```python
from build123d import *

# Parameters (mm, degrees)
F0_R     = 30
F0_R_2   = 4
F1_DEPTH = 12
F2_R     = 2.25
F3_DEPTH = 2
F4_R     = 1.55
F5_DEPTH = 25
F6_R     = 3
F7_DEPTH = 6
F9_DEPTH = 2
F10_SIZE = 0.5


with BuildPart() as f1:
    # F0 (on Top) → F1 (new body)
    with BuildSketch(Plane.XY):
        Circle(F0_R)
        Circle(F0_R_2, mode=Mode.SUBTRACT)
    extrude(amount=F1_DEPTH)

    # F2 (on face) → F3 (cut)
    with BuildSketch(Plane.XY.offset(12)):
        with Locations((0, 11.425)):
            Circle(F2_R)
    extrude(amount=-F3_DEPTH, mode=Mode.SUBTRACT)

    # F4 (on face) → F5 (cut)
    with BuildSketch(Plane.XY.offset(12)):
        with Locations((8.7, 20.925)):
            Circle(F4_R)
        with Locations((-8.7, 20.925)):
            Circle(F4_R)
        with Locations((0, -13.7)):
            Circle(F4_R)
    extrude(amount=-F5_DEPTH, mode=Mode.SUBTRACT)

    # F6 (on face) → F7 (cut)
    with BuildSketch(Plane(origin=(0, 0, 0), x_dir=(1, 0, 0), z_dir=(0, 0, -1))):
        with Locations((0, 13.7)):
            Circle(F6_R)
        with Locations((-8.7, -20.925)):
            Circle(F6_R)
        with Locations((8.7, -20.925)):
            Circle(F6_R)
    extrude(amount=-F7_DEPTH, mode=Mode.SUBTRACT)

    # F8 (on face) → F9 (cut)
    with BuildSketch(Plane.XY.offset(12)):
        with BuildLine():
            Line((21.28461, 11.133975), (26.466324, 14.125639))
            ThreePointArc((26.466324, 14.125639), (25.980762, 15), (25.466324, 15.85769))
            Line((25.466324, 15.85769), (20.28461, 12.866025))
            Line((20.28461, 12.866025), (21.28461, 11.133975))
        make_face()
        with BuildLine():
            Line((1, -29.983329), (1, -24))
            Line((1, -24), (-1, -24))
            Line((-1, -24), (-1, -29.983329))
            ThreePointArc((-1, -29.983329), (0, -30), (1, -29.983329))
        make_face()
        with BuildLine():
            Line((-20.28461, 12.866025), (-25.466324, 15.85769))
            ThreePointArc((-25.466324, 15.85769), (-25.980762, 15), (-26.466324, 14.125639))
            Line((-26.466324, 14.125639), (-21.28461, 11.133975))
            Line((-21.28461, 11.133975), (-20.28461, 12.866025))
        make_face()
    extrude(amount=-F9_DEPTH, mode=Mode.SUBTRACT)

    # F10
    f10_edges = [f1.edges().sort_by_distance(p)[0] for p in [
        (-30, 0, 0),
        (-3, -13.7, 0),
        (-4, 0, 0),
        (-11.7, 20.925, 0),
        (5.7, 20.925, 0),
    ]]
    chamfer(f10_edges, length=F10_SIZE)


solid = f1.part
```
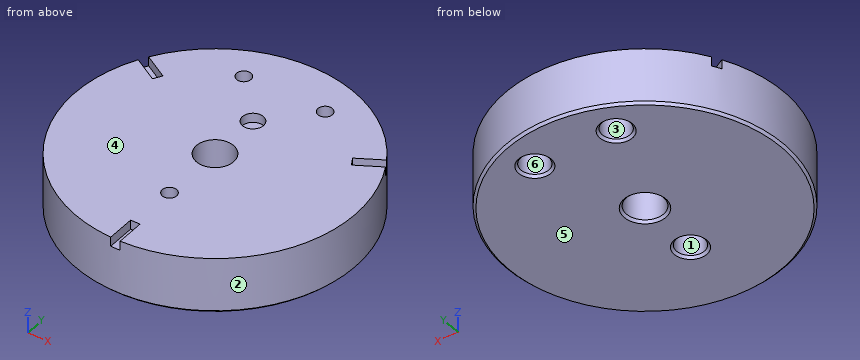
The listing builds one solid part. Answer for the finished solid, in the listing's coordinates (mm). Face numbers are marked on the shaded views. A direction names the side the tool comes from. Give positions to 0.01 mm unless a question says otherwise; leave off trailing zeros. Loops run counter-clockwise (first coordinate to the right, second up) from the corner with the lowest first, then second, coordinate; pieces in that order, holes last. Notation, with made-up numbers: (-16.75, -34) - (40.25, -34) arc R7 ccw to (40.25, -22) - close; hole circle Ø4 at (83.5, -35). An arc over 180 degrees is marked (long way). Return JSON: item names as keys, results as strings. Group by question number.
1. Find section C-C (z = 3.5). Write down the section's boundary in (x, y) (3 decimals), then the cut area to 3 significant figures.
2. Determine the mould class of the marked faces 1, 2, 3 and 4 for opening direction Y: pulls with the +Y half, pulls with the -Y half, needs draft (parallel to the pull), parting line crosses it, or undercut.
3. Given pin 1 Ø3 at (x, y) = (-10, 22) entering from -Z; pin 2 Ø0.6 at (x, y) = (0, -27.5) entering from +Z; pin 3 Ø4 at (x, y) = (23.5, 13.5) entering from +Z; pin 4 Ø1.5 at (x, z) = (-3.5, 2.5) entering from -Y, each flat-ended and moving along its own axis, determine where each tip first touches the part or whether it passes through.
4. Find section B-B (y = 0). Write down the section's boundary in (x, z).
5. Find section A-A (x = 0). Write down the section's boundary in (y, z) (3 decimals), then the cut area to 3 significant figures.
6. Which of the six approach directions +Z, -Z, +X, -X, +Y, -Y give full straight-line access (tool end or side, diameter ignored) to the marked faces 5 and 6?
7. Find section D-D (z = 8.75). Write down the section's boundary in (x, y) (3 decimals), then the cut area to 3 significant figures.
8. Straight lines are drawn through the part: line 1 (Y direction, x = 0, z = 5); line 2 (X direction, y = 20.5, z = 3.75); line 3 (X direction, y = -3.5, z = 1.25). For each, find the intervals that lie inside material, in ascending order. Write a range as [from, to].
Verdict:
{
 "1": {"outline": "circle Ø60 at (0, 0); hole circle Ø6 at (-8.7, 20.925); hole circle Ø8 at (0, 0); hole circle Ø6 at (0, -13.7); hole circle Ø6 at (8.7, 20.925)", "area": "2,690 mm^2"},
 "2": {"face 1": "undercut", "face 2": "parting line crosses it", "face 3": "undercut", "face 4": "needs draft"},
 "3": {"pin 1": "stops at z = 0.31", "pin 2": "stops at z = 10", "pin 3": "stops at z = 12", "pin 4": "stops at y = -29.87"},
 "4": {"outline": "(-30, 0.5) - (-29.5, 0) - (-4.5, 0) - (-4, 0.5) - (-4, 12) - (-30, 12) - close; (4, 0.5) - (4.5, 0) - (29.5, 0) - (30, 0.5) - (30, 12) - (4, 12) - close"},
 "5": {"outline": "(-30, 0.5) - (-29.5, 0) - (-17.2, 0) - (-16.7, 0.5) - (-16.7, 6) - (-15.25, 6) - (-15.25, 12) - (-24, 12) - (-24, 10) - (-30, 10) - close; (-12.15, 6) - (-10.7, 6) - (-10.7, 0.5) - (-10.2, 0) - (-4.5, 0) - (-4, 0.5) - (-4, 12) - (-12.15, 12) - close; (4, 0.5) - (4.5, 0) - (29.5, 0) - (30, 0.5) - (30, 12) - (13.675, 12) - (13.675, 10) - (9.175, 10) - (9.175, 12) - (4, 12) - close", "area": "548 mm^2"},
 "6": {"face 5": "-Z, +X, -X, +Y, -Y", "face 6": "-Z"},
 "7": {"outline": "circle Ø60 at (0, 0); hole circle Ø3.1 at (-8.7, 20.925); hole circle Ø8 at (0, 0); hole circle Ø3.1 at (0, -13.7); hole circle Ø3.1 at (8.7, 20.925)", "area": "2,750 mm^2"},
 "8": {"line 1": "y = [-30, -16.7], [-10.7, -4], [4, 30]", "line 2": "x = [-21.9, -11.67], [-5.73, 5.73], [11.67, 21.9]", "line 3": "x = [-29.8, -1.94], [1.94, 29.8]"}
}
